Geometry check sheet. Reference: drawing and pictorial views, mm from the part's lowest x, y, z. A direction names the side the tool comes from. Give positions to 0.01 mm unless a question says otherwise; leave off trailing zeros. Order: outer loops, then holes, each group sorted by start corner. A loop starts at its lowest first (then second) coordinate and runs counter-clockwise, first axis right, second up. Notation, with made-up numbers: (-15, 41) -> (11, 41) arc R17 ccw to (11, 47) -> close; hole circle Ø7 at (75.5, -24). An arc over 180 degrees is marked (long way). Write each question's results on one line, items separated by ' | '. Start each with the question number.
1. Mould release check, pull along Z, two halves, no side actions. Record for the marked faces 4, 5 and 6: +Z half, -Z half, draft (parallel to the pull), parting line (faces both ways), or undercut.
2. Cross-section at A-A, the plane y = 1.25. Enter the section's corners in (x, z).
3. Cross-section at B-B, the plane x = 4.25. Enter the section's corners in (y, z).
4. Material ranges on L1, parallel to Z at x = 4.25, y = 0.75; L2, parallel to Z at x = 4.75, y = 2; L3, parallel to Z at x = 15.5, y = 3.75, recorded low to high. Write a range as from..to.
5. Cross-section at C-C, the plane z = 22.3. Enter the section's corners in (x, y).
6. Depth check by flat-ended pin: pin 1 Ø0.8 at (y, z) = (1, 3.5) entering from +X; pin 2 Ø3 at (x, y) = (9, 5) entering from -Z; pin 3 Ø1.5 at (x, z) = (4.5, 2.5) entering from +Y. Enter the tip coordinate at first touch or a pass-through.
7. Set-up check for the marked faces 1, 2 and 3: record each of +Z, -Z, +X, -X, +Y, -Y from which the full face is reachable in a straight line by a thin tool's end or side.
8. Cross-section at D-D, the plane y = 8.5. Enter the section's corners in (x, z), then the cut area to 3 significant figures.
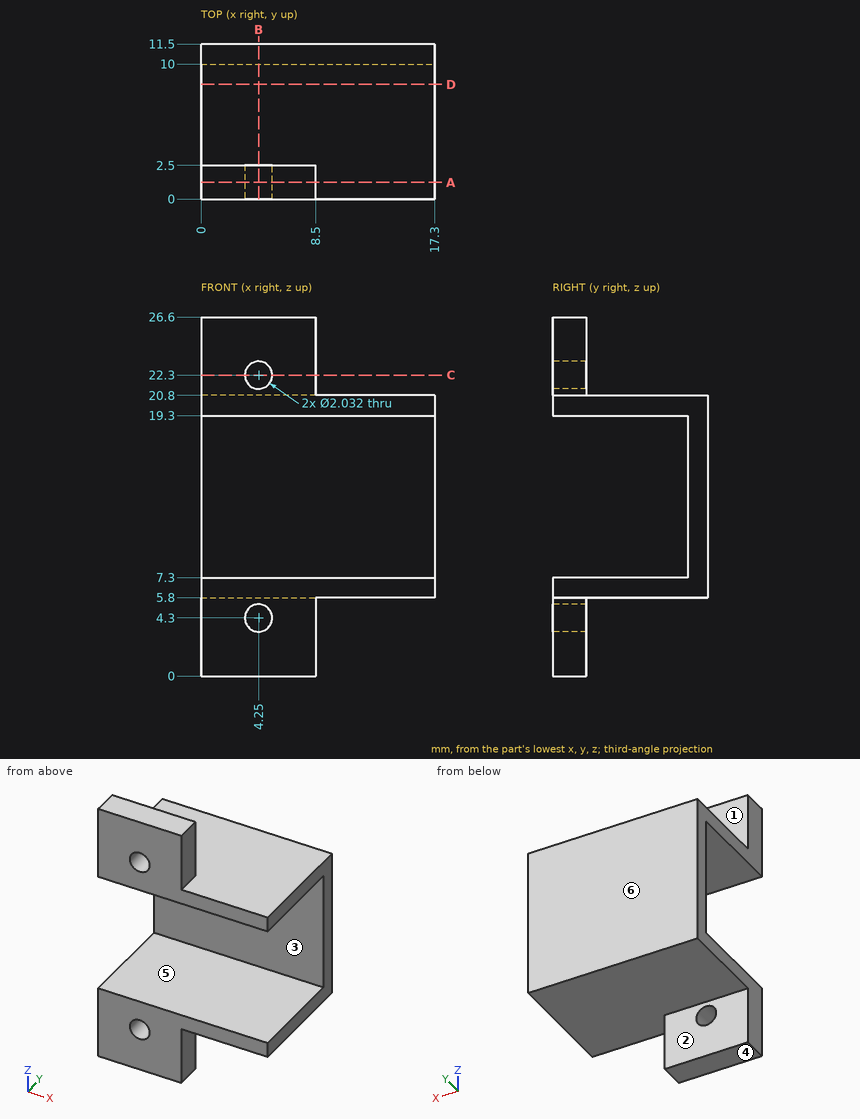
Results below:
1) face 4: -Z half | face 5: undercut | face 6: draft
2) outline: (0, 0) -> (8.5, 0) -> (8.5, 5.8) -> (17.3, 5.8) -> (17.3, 7.3) -> (0, 7.3) -> close; (0, 19.3) -> (17.3, 19.3) -> (17.3, 20.8) -> (8.5, 20.8) -> (8.5, 26.6) -> (0, 26.6) -> close; hole circle Ø2.03 at (4.25, 4.3); hole circle Ø2.03 at (4.25, 22.3)
3) outline: (0, 0) -> (2.5, 0) -> (2.5, 3.28) -> (0, 3.28) -> close; (0, 5.32) -> (2.5, 5.32) -> (2.5, 5.8) -> (11.5, 5.8) -> (11.5, 20.8) -> (2.5, 20.8) -> (2.5, 21.28) -> (0, 21.28) -> (0, 19.3) -> (10, 19.3) -> (10, 7.3) -> (0, 7.3) -> close; (0, 23.32) -> (2.5, 23.32) -> (2.5, 26.6) -> (0, 26.6) -> close
4) L1: z = 0..3.28, 5.32..7.3, 19.3..21.28, 23.32..26.6 | L2: z = 0..3.42, 5.18..7.3, 19.3..21.42, 23.18..26.6 | L3: z = 5.8..7.3, 19.3..20.8
5) outline: (0, 0) -> (3.23, 0) -> (3.23, 2.5) -> (0, 2.5) -> close; (5.27, 0) -> (8.5, 0) -> (8.5, 2.5) -> (5.27, 2.5) -> close
6) pin 1: stops at x = 8.5 | pin 2: stops at z = 5.8 | pin 3: stops at y = 2.5
7) face 1: +Z, +X, -X, +Y | face 2: -Z, +X, -X, +Y | face 3: +X, -X, -Y
8) outline: (0, 5.8) -> (17.3, 5.8) -> (17.3, 7.3) -> (0, 7.3) -> close; (0, 19.3) -> (17.3, 19.3) -> (17.3, 20.8) -> (0, 20.8) -> close | area: 51.9 mm²
